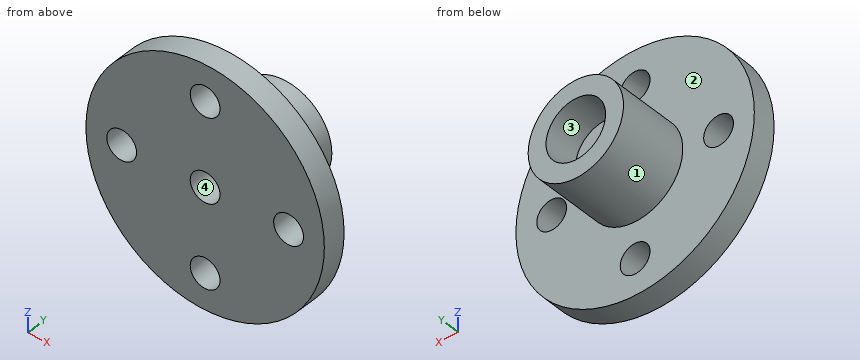
from build123d import *

# Parameters (mm, degrees)
SKETCH1_R                       = 10
BOSS_EXTRUDE1_DEPTH             = 2
TAP_DRILL_FOR_M3X0_5_TAP1_D     = 2.5
TAP_DRILL_FOR_M3X0_5_TAP1_DEPTH = 38.1
CIRPATTERN1_COUNT               = 4
SKETCH4_R                       = 4
BOSS_EXTRUDE2_DEPTH             = 6
SKETCH5_R                       = 2.5
CUT_EXTRUDE1_DEPTH              = 3
TAP_DRILL_FOR_M3X0_5_TAP2_D     = 2.5
TAP_DRILL_FOR_M3X0_5_TAP2_DEPTH = 38.1


with BuildPart() as part:
    # Sketch1 → Boss-Extrude1 (new body)
    with BuildSketch(Plane(origin=(0, 0, 0), x_dir=(1, 0, 0), z_dir=(0, 1, 0))):
        Circle(SKETCH1_R)
    extrude(amount=BOSS_EXTRUDE1_DEPTH)

    # Tap Drill for M3x0.5 Tap1
    with Locations(Plane(origin=(0, 2, 0), x_dir=(1, 0, 0), z_dir=(0, 1, 0))):
        with Locations((7, 0)):
            tap_drill_for_m3x0_5_tap1 = Hole(TAP_DRILL_FOR_M3X0_5_TAP1_D / 2, depth=TAP_DRILL_FOR_M3X0_5_TAP1_DEPTH)

    # CirPattern1: Tap Drill for M3x0.5 Tap1 ×4 about axis
    cirpattern1_axis = Axis((0, 0, 0), (0, 1, 0))
    for i in range(1, CIRPATTERN1_COUNT):
        add(tap_drill_for_m3x0_5_tap1.rotate(cirpattern1_axis, i * 360 / CIRPATTERN1_COUNT), mode=Mode.SUBTRACT)

    # Sketch4 → Boss-Extrude2 (add)
    with BuildSketch(Plane(origin=(0, 2, 0), x_dir=(1, 0, 0), z_dir=(0, 1, 0))):
        Circle(SKETCH4_R)
    extrude(amount=BOSS_EXTRUDE2_DEPTH)

    # Sketch5 → Cut-Extrude1 (cut)
    with BuildSketch(Plane(origin=(0, 8, 0), x_dir=(1, 0, 0), z_dir=(0, 1, 0))):
        Circle(SKETCH5_R)
    extrude(amount=-CUT_EXTRUDE1_DEPTH, mode=Mode.SUBTRACT)

    # Tap Drill for M3x0.5 Tap2
    with Locations(Plane(origin=(0, 5, 0), x_dir=(1, 0, 0), z_dir=(0, 1, 0))):
        with Locations((0, 0)):
            Hole(TAP_DRILL_FOR_M3X0_5_TAP2_D / 2, depth=TAP_DRILL_FOR_M3X0_5_TAP2_DEPTH)


solid = part.part
Can you work these out from the model? Positions are in its coordinate system, mm. Face numbers are marked on the shaded views. Coordinates: 2 decimals unless noted, no trailing zeros. Loops run counter-clockwise (first coordinate to the right, second up) from the corner with the lowest first, then second, coordinate; pieces in that order, holes last. Notation, with made-up numbers: (4.5, 37.5) - (49.5, 37.5) arc R35 ccw to (49.5, 71.5) - close; hole circle Ø11 at (-21.75, 0). An arc over 180 degrees is marked (long way). Put each result on its own line as item: value. Start each with the question number.
Item 1: Suppose I cut it at A-A (z = 0). Please give me the cut outline in (x, y).
Item 2: If we mould it in two halves opening along X, with no side actions, what happens to the marked faces 1, 2, 3 and 4? For each: +X half, -X half, draft (parallel to the pull), parting line (faces both ways), or undercut.
Item 3: For pin 1 (1 mm diameter, centred on y = 3, z = 2, fed in from +X); pin 2 (1.5 mm diameter, centred on x = 0, z = 7, fed in from +Y); pin 3 (3 mm diameter, centred on x = -7, z = 0, fed in from +Y); pin 4 (1 mm diameter, centred on x = -1.5, y = 7, fed in from +Z), each with a flat end and sliding along its axis, tell me the tip position at first contact or that it passes through.
Item 4: Suppose I cut it at D-D (x = 0.75). Please give me the cut outline in (y, z), and give its area (3 significant figures).
Item 5: If I drill on line 1 along Z through (x, y) = (0, 2.3); line 2 along Z through (x, y) = (0, 6.05); line 3 along Y through (x, z) = (7, 2.25), over which ranges is the centre line in solid material (lowest first)?
Item 6: Suppose I cut it at B-B (x = -7). Please give me the cut outline in (y, z), and give its area (3 significant figures).
Item 7: Suppose I cut it at C-C (z = -6.5). Please give me the cut outline in (x, y).
Here are the results:
1. outline: (-10, 0) - (-8.25, 0) - (-8.25, 2) - (-10, 2) - close; (-5.75, 0) - (-1.25, 0) - (-1.25, 5) - (-2.5, 5) - (-2.5, 8) - (-4, 8) - (-4, 2) - (-5.75, 2) - close; (1.25, 0) - (5.75, 0) - (5.75, 2) - (4, 2) - (4, 8) - (2.5, 8) - (2.5, 5) - (1.25, 5) - close; (8.25, 0) - (10, 0) - (10, 2) - (8.25, 2) - close
2. face 1: parting line
2. face 2: draft
2. face 3: undercut
2. face 4: undercut
3. pin 1: x = 3.71
3. pin 2: through
3. pin 3: y = 2
3. pin 4: z = 3.87
4. outline: (0, -9.97) - (2, -9.97) - (2, -8) - (0, -8) - close; (0, -6) - (2, -6) - (2, -3.93) - (8, -3.93) - (8, -2.38) - (5, -2.38) - (5, -1) - (0, -1) - close; (0, 1) - (5, 1) - (5, 2.38) - (8, 2.38) - (8, 3.93) - (2, 3.93) - (2, 6) - (0, 6) - close; (0, 8) - (2, 8) - (2, 9.97) - (0, 9.97) - close
4. area: 54.7 mm²
5. line 1: -4 to -1.25, 1.25 to 4
5. line 2: -4 to -2.5, 2.5 to 4
5. line 3: 0 to 2
6. outline: (0, -7.14) - (2, -7.14) - (2, -1.25) - (0, -1.25) - close; (0, 1.25) - (2, 1.25) - (2, 7.14) - (0, 7.14) - close
6. area: 23.6 mm²
7. outline: (-7.6, 0) - (-1.15, 0) - (-1.15, 2) - (-7.6, 2) - close; (1.15, 0) - (7.6, 0) - (7.6, 2) - (1.15, 2) - close
